Build history of the part. All positions in model axes, mm. Face numbers are marked on the shaded views. A direction names the side the tool comes from. Give positions to 0.01 mm unless a question says otherwise; leave off trailing zeros. Loops run counter-clockwise (first coordinate to the right, second up) from the corner with the lowest first, then second, coordinate; pieces in that order, holes last. Notation, with made-up numbers: (-6, -22) -> (22, -22) arc R18 ccw to (22, 12) -> close; hole circle Ø6 at (-25.5, -15.75). An arc over 180 degrees is marked (long way). Answer as a JSON object with one key per item and string values. Group by question number.
Q1. Band-saw the part on D-D, the plane y = -62. Write the cut outline in (x, z).
Q2. Band-saw the part on A-A, the plane x = 4.66. Write the cut outline in (y, z), plus the area to 3 significant figures.
Q3. Two-plate mould, pull along Y, no slides. Class the marked faces 1, 2, 3 and 4: pulls with the +Y half, pulls with the -Y half, needs draft (parallel to the pull), parting line crosses it, or undercut.
Q4. Wall check: probe 1 along X at (y, z) = (-2, 10.5); probe 2 along Y at (x, z) = (4.66, -6.5); probe 3 along Y at (x, z) = (-14, 10). Give the ranges that are in metal, low to high. Write a range as from..to.
Q5. Tool access for the marked faces 5 and 6: list every direction of +Z, -Z, +X, -X, +Y, -Y with a clear straight run to the whole face (end or side of a thin tool).
Q6. Band-saw the part on B-B, the plane y = -7.02. Write the cut outline in (x, z).
Q7. Drop flat-ended pins along their axis: pin 1 (14.5 mm diameter, centred on y = 25, z = 12.5, fed in from +X); pin 2 (4.5 mm diameter, centred on x = -10.93, y = -25.02, fed in from +Z); pin 3 (4 mm diameter, centred on x = 45, y = -24, fed in from +Z). Give the stop position or say it passes through.
Q8. Band-saw the part on C-C, the plane y = 25.48. Write the cut outline in (x, z), plus the area to 3 significant figures.
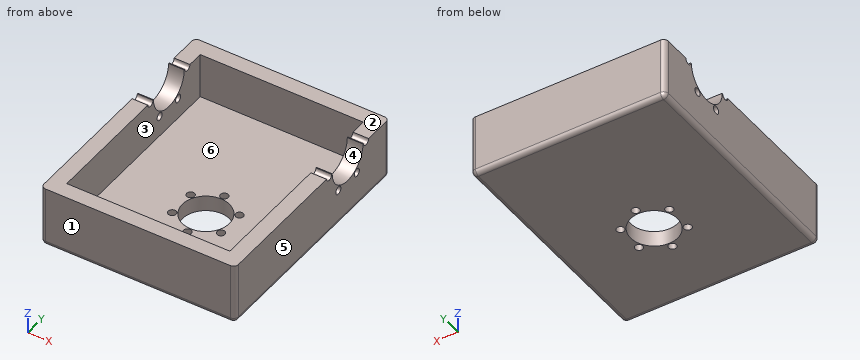
from build123d import *

# Parameters (mm, degrees)
SKETCH1_W               = 124
SKETCH1_H               = 150
SKETCH1_W_2             = 104
SKETCH1_H_2             = 130
BOSS_EXTRUDE1_DEPTH     = 29
SKETCH2_W               = 124
SKETCH2_H               = 150
BOSS_EXTRUDE2_DEPTH     = 10
CUT_EXTRUDE1_DEPTH      = 105.833200848
CUT_EXTRUDE1_DEPTH_BACK = 105.833200848
SKETCH3_R               = 15
SKETCH3_R_2             = 2.5
CUT_EXTRUDE2_DEPTH      = 148.79039211
CUT_EXTRUDE2_DEPTH_BACK = 148.79039211
SKETCH4_R               = 15
SKETCH4_R_2             = 2.5
FILLET1_R               = 3


with BuildPart() as part:
    # Sketch1 → Boss-Extrude1 (new body)
    with BuildSketch(Plane.XY):
        Rectangle(SKETCH1_W, SKETCH1_H)
        Rectangle(SKETCH1_W_2, SKETCH1_H_2, mode=Mode.SUBTRACT)
    extrude(amount=BOSS_EXTRUDE1_DEPTH)

    # Sketch2 → Boss-Extrude2 (add)
    with BuildSketch(Plane(origin=(0, 0, 0), x_dir=(-1, 0, 0), z_dir=(0, 0, -1))):
        Rectangle(SKETCH2_W, SKETCH2_H)
    extrude(amount=BOSS_EXTRUDE2_DEPTH)

    # Sketch3 → Cut-Extrude1 (cut, two sides: drawn at the far end of the back side and taken through both)
    with BuildSketch(Plane(origin=(0, 0, -10), x_dir=(-1, 0, 0), z_dir=(0, 0, -1)).offset(-CUT_EXTRUDE1_DEPTH_BACK)):
        with Locations(Location((-4.66, -16.02, 0), (0, 0, 180))):
            Circle(SKETCH3_R)
        with Locations(Location((-4.66, 1.98, 0), (0, 0, 180))):
            Circle(SKETCH3_R_2)
        with Locations(Location((10.928457268, -7.02, 0), (0, 0, 180))):
            Circle(SKETCH3_R_2)
        with Locations(Location((10.928457268, -25.02, 0), (0, 0, 180))):
            Circle(SKETCH3_R_2)
        with Locations(Location((-4.66, -34.02, 0), (0, 0, 180))):
            Circle(SKETCH3_R_2)
        with Locations(Location((-20.248457268, -25.02, 0), (0, 0, 180))):
            Circle(SKETCH3_R_2)
        with Locations(Location((-20.248457268, -7.02, 0), (0, 0, 180))):
            Circle(SKETCH3_R_2)
    extrude(amount=CUT_EXTRUDE1_DEPTH + CUT_EXTRUDE1_DEPTH_BACK, mode=Mode.SUBTRACT)

    # Sketch4 → Cut-Extrude2 (cut, two sides: drawn at the far end of the back side and taken through both)
    with BuildSketch(Plane.ZY.offset(62).offset(-CUT_EXTRUDE2_DEPTH_BACK)):
        with Locations((29, 34.48)):
            Circle(SKETCH4_R)
        with Locations((29, 52.48)):
            Circle(SKETCH4_R_2)
        with Locations((44.588457268, 43.48)):
            Circle(SKETCH4_R_2)
        with Locations((44.588457268, 25.48)):
            Circle(SKETCH4_R_2)
        with Locations((29, 16.48)):
            Circle(SKETCH4_R_2)
        with Locations(Location((13.411542732, 25.48, 0), (0, 0, 270))):
            Circle(SKETCH4_R_2)
        with Locations(Location((13.411542732, 43.48, 0), (0, 0, 270))):
            Circle(SKETCH4_R_2)
    extrude(amount=CUT_EXTRUDE2_DEPTH + CUT_EXTRUDE2_DEPTH_BACK, mode=Mode.SUBTRACT)

    # Fillet1
    fillet1_edges = [part.edges().sort_by_distance(p)[0] for p in [
        (0, 75, -10),
        (62, 0, -10),
        (0, -75, -10),
        (-62, 0, -10),
        (62, -75, 9.5),
        (-62, -75, 9.5),
        (-62, 75, 9.5),
        (62, 75, 9.5),
    ]]
    fillet(fillet1_edges, radius=FILLET1_R)


solid = part.part
Worked answers:
{
 "1": {"outline": "(-62, -7) arc R3 ccw to (-59, -10) -> (59, -10) arc R3 ccw to (62, -7) -> (62, 29) -> (52, 29) -> (52, 0) -> (-52, 0) -> (-52, 29) -> (-62, 29) -> close"},
 "2": {"outline": "(-75, -7) arc R3 ccw to (-72, -10) -> (-36.52, -10) -> (-36.52, 0) -> (-65, 0) -> (-65, 29) -> (-75, 29) -> close; (-31.52, -10) -> (-31.02, -10) -> (-31.02, 0) -> (-31.52, 0) -> close; (-1.02, -10) -> (-0.52, -10) -> (-0.52, 0) -> (-1.02, 0) -> close; (4.48, -10) -> (72, -10) arc R3 ccw to (75, -7) -> (75, 29) -> (65, 29) -> (65, 0) -> (4.48, 0) -> close", "area": "1,680 mm2"},
 "3": {"face 1": "pulls with the -Y half", "face 2": "needs draft", "face 3": "undercut", "face 4": "undercut"},
 "4": {"probe 1": "-62..-52, 52..62", "probe 2": "-75..-36.52, -31.52..-31.02, -1.02..-0.52, 4.48..75", "probe 3": "-75..-65, 65..75"},
 "5": {"face 5": "+Z, -Z, +X, +Y, -Y", "face 6": "+Z"},
 "6": {"outline": "(-62, -7) arc R3 ccw to (-59, -10) -> (-13.43, -10) -> (-13.43, 0) -> (-52, 0) -> (-52, 29) -> (-62, 29) -> close; (-8.43, -10) -> (-7.34, -10) -> (-7.34, 0) -> (-8.43, 0) -> close; (16.66, -10) -> (17.75, -10) -> (17.75, 0) -> (16.66, 0) -> close; (22.75, -10) -> (59, -10) arc R3 ccw to (62, -7) -> (62, 29) -> (52, 29) -> (52, 0) -> (22.75, 0) -> close"},
 "7": {"pin 1": "x = 62", "pin 2": "through", "pin 3": "z = 0"},
 "8": {"outline": "(-62, -7) arc R3 ccw to (-59, -10) -> (59, -10) arc R3 ccw to (62, -7) -> (62, 10.91) -> (52, 10.91) -> (52, 0) -> (-52, 0) -> (-52, 10.91) -> (-62, 10.91) -> close; (-62, 15.91) -> (-52, 15.91) -> (-52, 17) -> (-62, 17) -> close; (52, 15.91) -> (62, 15.91) -> (62, 17) -> (52, 17) -> close", "area": "1,480 mm2"}
}
